Check sheet for the modelled part. Datum: model origin and axes. Units: mm. A direction names the side the tool comes from. Coordinates: 2 decimals unless noted, no trailing zeros. Loops run counter-clockwise (first coordinate to the right, second up) from the corner with the lowest first, then second, coordinate; pieces in that order, holes last. Notation, with made-up numbers: (-38.5, 64) -> (-2.5, 64) arc R23 cw to (-2.5, 102) -> close; hole circle Ø6 at (-14, 89.5). An arc over 180 degrees is marked (long way). Use CSV: the item, a comma, the result in double quotes.
```python
from build123d import *

# Parameters (mm, degrees)
F0_R      = 7.874
F1_DEPTH  = 15.748
F2_W      = 57.912
F2_H      = 50.8
F3_DEPTH  = 3.048
F3_FACE_W = 57.912
F3_FACE_H = 50.8
F4_DEPTH  = 25.4
F5_R      = 28.956
F6_DEPTH  = 50.8
F8_DEPTH  = 50.8
F10_DEPTH = 177.8


with BuildPart() as f1:
    # F0 (on Top) → F1 (new body)
    with BuildSketch(Plane.XY):
        Polygon((13.202934, 3.150654), (-53.345066, 3.150654), (-53.345066, -47.649346), (13.202934, -47.649346), (13.202934, -22.249346), align=None)
        with Locations((-34.549066, -22.249346)):
            Circle(F0_R, mode=Mode.SUBTRACT)
        with BuildLine():
            ThreePointArc((68.828934, -22.249346), (60.954934, -14.375346), (53.080934, -22.249346))
            ThreePointArc((53.080934, -22.249346), (60.954934, -30.123346), (68.828934, -22.249346))
        make_face()
        Polygon((79.750934, 3.150654), (13.202934, 3.150654), (13.202934, -22.249346), (13.202934, -47.649346), (79.750934, -47.649346), align=None)
        with BuildLine():
            ThreePointArc((68.828934, -22.249346), (60.954934, -30.123346), (53.080934, -22.249346))
            ThreePointArc((53.080934, -22.249346), (60.954934, -14.375346), (68.828934, -22.249346))
        make_face(mode=Mode.SUBTRACT)
    extrude(amount=F1_DEPTH)

    # F2 (on face) → F3 (join)
    with BuildSketch(Plane.XY.offset(15.748)):
        with Locations((13.202934, -22.249346)):
            Rectangle(F2_W, F2_H)
    extrude(amount=F3_DEPTH)

    # F3_face (on face) → F4 (join)
    with BuildSketch(Plane(origin=(13.202934, -22.249346, 18.796), x_dir=(1, 0, 0), z_dir=(0, 0, 1))):
        Rectangle(F3_FACE_W, F3_FACE_H)
    extrude(amount=F4_DEPTH)

    # F5 (on face) → F6 (join)
    with BuildSketch(Plane.XZ.offset(47.649346)):
        with Locations((13.202934, 44.196)):
            Circle(F5_R)
    extrude(amount=-F6_DEPTH)

    # F7 (on face) → F8 (cut)
    with BuildSketch(Plane.XZ.offset(47.649346)):
        with BuildLine():
            ThreePointArc((13.202934, 61.976), (3.145047, 37.694113), (27.426934, 47.752))
            ThreePointArc((27.426934, 47.752), (23.260821, 57.809887), (13.202934, 61.976))
        make_face()
    extrude(amount=-F8_DEPTH, mode=Mode.SUBTRACT)

    # F9 (on face) → F10 (cut)
    with BuildSketch(Plane.YZ.offset(42.158934)):
        Polygon((-47.649346, 73.572527), (-47.649346, 15.748), (-26.602939, 73.572527), align=None)
    extrude(amount=-F10_DEPTH, mode=Mode.SUBTRACT)


solid = f1.part
```
1) Thickness scan on line 1 along Z through (x, y) = (-30, -6); line 2 along X through (y, z) = (-2, 19.5); line 3 along X through (y, z) = (-17.5, 42). Record the ranges inside material, lowest first. Write a range as from..to.
Answer below:
line 1,"z = 0..15.75"
line 2,"x = -15.75..42.16"
line 3,"x = -15.75..0.19, 26.21..42.16"
2) Cross-section at B-B on z = 35. Record the boundary of the cut face in (x, y), and give its area (3 significant figures).
Answer below:
outline,"(-15.75, -40.64) -> (6.9, -40.64) -> (6.9, 3.15) -> (-15.75, 3.15) -> close; (19.5, -40.64) -> (42.16, -40.64) -> (42.16, 3.15) -> (19.5, 3.15) -> close"
area,"1,980 mm²"
3) Access from +Z, -Z, +X, -X, +Y, -Y to the whole of each face (thin tool, end or side, straight path). Record for faces 1 (the flat face through (42.159, -23, 30)), 2 (the cylindrical face through (13.84, -12.861, 73.145)), 3 (the flat face through (-15.753, -23, 30)).
Answer below:
face 1,"+Z, +X, +Y, -Y"
face 2,"+Z, +Y, -Y"
face 3,"+Z, -X, +Y, -Y"
4) Cross-section at C-C on x = -33. Record the boundary of the cut face in (y, z), and give its area (3 significant figures).
Answer below:
outline,"(-47.65, 0) -> (-29.97, 0) -> (-29.97, 15.75) -> (-47.65, 15.75) -> close; (-14.53, 0) -> (3.15, 0) -> (3.15, 15.75) -> (-14.53, 15.75) -> close"
area,"557 mm²"
5) Cross-section at D-D on z = 7. Record the boundary of the cut face in (x, y), and give its area (3 significant figures).
Answer below:
outline,"(-53.35, -47.65) -> (79.75, -47.65) -> (79.75, 3.15) -> (-53.35, 3.15) -> close; hole circle Ø15.75 at (-34.55, -22.25); hole circle Ø15.75 at (60.95, -22.25)"
area,"6,370 mm²"
6) Go/stop test with flat-tipped pins: pin 1 Ø19 at (x, y) = (-43, -23) entering from +Z; pin 2 Ø6 at (x, y) = (-9, -17.5) entering from -Z; pin 3 Ø1.5 at (y, z) = (-5.5, 24.5) entering from -X; pin 4 Ø2 at (x, z) = (-13, 39) entering from -Y. Record where each tip stops, or that it passes through.
Answer below:
pin 1,"stops at z = 15.75"
pin 2,"stops at z = 0"
pin 3,"stops at x = -15.75"
pin 4,"stops at y = -39.55"
7) Draft check along Y on faces 4 (the flat face through (79.751, -23, 8)), 5 (the flat face through (12, 3.151, 29)), 6 (the cylindrical face through (53.445, -19.884, 7.764)), 7 (the flat face through (13.608, -41.992, 31.292)). Enter one of: released by +Y, released by -Y, zero draft, split by the parting line, or undercut.
Answer below:
face 4,"zero draft"
face 5,"released by +Y"
face 6,"undercut"
face 7,"released by -Y"
